Verification items for the finished model (mm, model axes). Face numbers are marked on the shaded views. A direction names the side the tool comes from. Round coordinates to 2 decimals unless told otherwise and drop trailing zeros. Order: outer loops, then holes, each group sorted by start corner. A loop starts at its lowest first (then second) coordinate and runs counter-clockwise, first axis right, second up. Notation, with made-up numbers: (46.25, 32.5) -> (84.25, 32.5) arc R19 ccw to (84.25, 51.5) -> close; hole circle Ø5 at (48.25, -8.5). An arc over 180 degrees is marked (long way). Put each result on its own line as item: value.
from build123d import *

# Parameters (mm, degrees)
BOSS_EXTRUDE1_DEPTH = 19
SKETCH2_R           = 1.8
CUT_EXTRUDE1_DEPTH  = 27.191601707
SKETCH2_3_R         = 3
SKETCH2_3_R_2       = 1.8
CUT_EXTRUDE2_DEPTH  = 12


with BuildPart() as part:
    # Sketch1 → Boss-Extrude1 (new body)
    with BuildSketch(Plane.XY):
        with BuildLine():
            Line((-10, 0), (-10, 15))
            Line((-10, 15), (10, 15))
            Line((10, 15), (10, 0))
            Line((10, 0), (3, 0))
            Line((3, 0), (3, 7))
            ThreePointArc((3, 7), (0, 10), (-3, 7))
            Line((-3, 7), (-3, 0))
            Line((-3, 0), (-10, 0))
        make_face()
    extrude(amount=BOSS_EXTRUDE1_DEPTH)

    # Sketch2 → Cut-Extrude1 (cut, through all)
    with BuildSketch(Plane(origin=(0, 15, 0), x_dir=(1, 0, 0), z_dir=(0, 1, 0))):
        with Locations(Location((-6.5, -9.5, 0), (0, 0, 270))):
            Circle(SKETCH2_R)
        with Locations(Location((6.5, -9.5, 0), (0, 0, 270))):
            Circle(SKETCH2_R)
    extrude(amount=-CUT_EXTRUDE1_DEPTH, mode=Mode.SUBTRACT)

    # Sketch2<3> → Cut-Extrude2 (cut)
    # profile 1 of 2: a face of its own
    with BuildSketch(Plane(origin=(0, 15, 0), x_dir=(1, 0, 0), z_dir=(0, 1, 0))):
        with Locations(Location((-6.5, -9.5, 0), (0, 0, 270))):
            Circle(SKETCH2_3_R)
        with Locations(Location((-6.5, -9.5, 0), (0, 0, 270))):
            Circle(SKETCH2_3_R_2, mode=Mode.SUBTRACT)
    # profile 2 of 2: a face of its own
    with BuildSketch(Plane(origin=(0, 15, 0), x_dir=(1, 0, 0), z_dir=(0, 1, 0))):
        with Locations(Location((6.5, -9.5, 0), (0, 0, 270))):
            Circle(SKETCH2_3_R)
        with Locations(Location((6.5, -9.5, 0), (0, 0, 270))):
            Circle(SKETCH2_3_R_2, mode=Mode.SUBTRACT)
    extrude(amount=-CUT_EXTRUDE2_DEPTH, mode=Mode.SUBTRACT)


solid = part.part
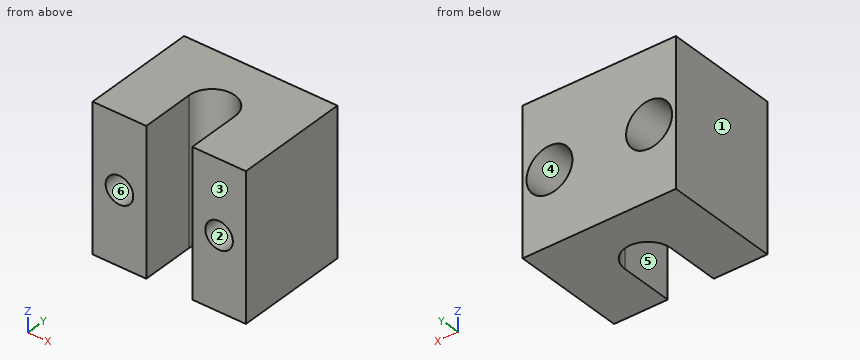
Item 1: Release check for a two-part mould opening along X. For the marked faces 1, 2 and 3 record: +X half, -X half, draft (parallel to the pull), parting line (faces both ways), or undercut.
Check sheet entries:
face 1: -X half
face 2: undercut
face 3: draft
Item 2: Material ranges on L1, parallel to X at y = 1.15, z = 9.5; L2, parallel to X at y = 12, z = 8; L3, parallel to X at y = 5.25, z = 4.5, recorded low to high. Write a range as [from, to].
Check sheet entries:
L1: x = [-10, -8.3], [-4.7, -3], [3, 4.7], [8.3, 10]
L2: x = [-10, -9.1], [-3.9, 3.9], [9.1, 10]
L3: x = [-10, -3], [3, 10]
Item 3: Section check A-A on y = 6. Record the boundary of the cut face in (x, z).
Check sheet entries:
outline: (-10, 0) -> (-3, 0) -> (-3, 19) -> (-10, 19) -> close; (3, 0) -> (10, 0) -> (10, 19) -> (3, 19) -> close; hole circle Ø6 at (-6.5, 9.5); hole circle Ø6 at (6.5, 9.5)
Item 4: Section check B-B on z = 9.5. Record the boundary of the cut face in (x, y), then the cut area to 3 significant figures.
Check sheet entries:
outline: (-10, 0) -> (-8.3, 0) -> (-8.3, 3) -> (-9.5, 3) -> (-9.5, 15) -> (-10, 15) -> close; (-4.7, 0) -> (-3, 0) -> (-3, 7) arc R3 cw to (3, 7) -> (3, 0) -> (4.7, 0) -> (4.7, 3) -> (3.5, 3) -> (3.5, 15) -> (-3.5, 15) -> (-3.5, 3) -> (-4.7, 3) -> close; (8.3, 0) -> (10, 0) -> (10, 15) -> (9.5, 15) -> (9.5, 3) -> (8.3, 3) -> close
area: 78.3 mm^2
Item 5: Tool access check on the marked faces 4, 5 and 6. Record the directions out of +Z, -Z, +X, -X, +Y, -Y that give a thin tool (end or side, any length) a straight path to the whole face; none if there is none.
Check sheet entries:
face 4: +Y
face 5: +Z, -Z, -Y
face 6: +Y, -Y
Item 6: Section check D-D on z = 1.5. Record the boundary of the cut face in (x, y), then the cut area to 3 significant figures.
Check sheet entries:
outline: (-10, 0) -> (-3, 0) -> (-3, 7) arc R3 cw to (3, 7) -> (3, 0) -> (10, 0) -> (10, 15) -> (-10, 15) -> close
area: 244 mm^2
Item 7: Section check C-C on x = -6.5. Record the boundary of the cut face in (y, z), then the cut area to 3 significant figures.
Check sheet entries:
outline: (0, 0) -> (15, 0) -> (15, 6.5) -> (3, 6.5) -> (3, 7.7) -> (0, 7.7) -> close; (0, 11.3) -> (3, 11.3) -> (3, 12.5) -> (15, 12.5) -> (15, 19) -> (0, 19) -> close
area: 202 mm^2
Item 8: Gauge pin test, flat end, axial feed: pin 1 Ø3 at (x, z) = (-7, 8.5) entering from +Y. Record the tip position at first contact, or that the pin passes through.
Check sheet entries:
pin 1: stops at y = 3
